from build123d import *

# Parameters (mm, degrees)
F0_W     = 101.6
F0_H     = 76.2
F0_W_2   = 95.25
F0_H_2   = 69.85
F1_DEPTH = 130
F2_W     = 250
F2_H     = 35
F3_DEPTH = 3.175


with BuildPart() as f1:
    # F0 (on Right) → F1 (new body, symmetric)
    with BuildSketch(Plane.YZ):
        Rectangle(F0_W, F0_H)
        Rectangle(F0_W_2, F0_H_2, mode=Mode.SUBTRACT)
    extrude(amount=F1_DEPTH, both=True)

    # F2 (on face) → F3 (cut, through all)
    with BuildSketch(Plane.XZ.offset(50.8)):
        with Locations((0, -15.6)):
            Rectangle(F2_W, F2_H)
    extrude(amount=-F3_DEPTH, mode=Mode.SUBTRACT)


solid = f1.part
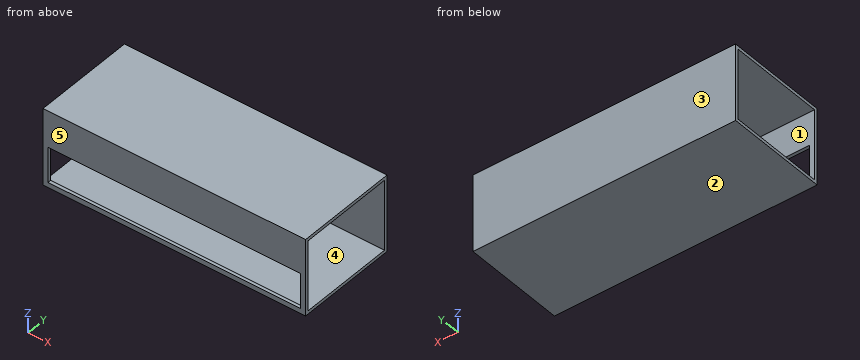
The model under review builds one solid part; all positions refer to its coordinate system, in mm. Face numbers are marked on the shaded views. A direction names the side the tool comes from. Coordinates: 2 decimals unless noted, no trailing zeros. Write each loop counter-clockwise with the first axis right and the second up, starting at its lowest first coordinate (ties: lowest second). Pieces come first, ordered by that corner, then holes. Notation, with made-up numbers: (72.25, 15) - (109.25, 15) arc R35 ccw to (109.25, 52) - close; hole circle Ø9 at (-27.75, -4). An arc over 180 degrees is marked (long way). Answer as a JSON object with one key per item and string values. Group by question number.
1. Add section A-A (z = -16). Give the boundary of the cut face in (x, y) (3 decimals), plus the area to 3 significant figures.
2. Add section D-D (x = 13). Give the boundary of the cut face in (y, z) (3 decimals), plus the area to 3 significant figures.
3. Clearance check with a flat-ended pin moving along its axis: pin 1 Ø10 at (x, z) = (-40.5, -24) entering from -Y (3 decimals). State where the tip first meets the part, or that it passes through.
4. Machinability: for the marked faces 4 and 5, which of the approach directions +Z, -Z, +X, -X, +Y, -Y give a long, thin tool a straight path to every point of the face, cutting with its end or side? Answer none if there is none.
5. To check wall thickness, follow probe 1 along Z at (x, y) = (-11, 14.5) (3 decimals); probe 2 along Y at (x, z) = (-26.5, 15) (3 decimals); probe 3 along Y at (x, z) = (17, -15) (3 decimals). State the ranges of each line that lie inside material, in increasing order.
6. Mouldability with a two-part tool opening along Y and no side actions: class the marked faces 1, 2 and 3 as pulls with the +Y half, pulls with the -Y half, needs draft (parallel to the pull), parting line crosses it, or undercut.
7. Add section B-B (y = -23.5). Give the boundary of the cut face in (x, z) (3 decimals), plus the area to 3 significant figures.
8. Add section C-C (z = 20.5). Give the boundary of the cut face in (x, y) (3 decimals).
Findings:
{
 "1": {"outline": "(-130, -50.8) - (-125, -50.8) - (-125, -47.625) - (-130, -47.625) - close; (-130, 47.625) - (130, 47.625) - (130, 50.8) - (-130, 50.8) - close; (125, -50.8) - (130, -50.8) - (130, -47.625) - (125, -47.625) - close", "area": "857 mm²"},
 "2": {"outline": "(-50.8, -38.1) - (50.8, -38.1) - (50.8, 38.1) - (-50.8, 38.1) - (-50.8, 1.9) - (-47.625, 1.9) - (-47.625, 34.925) - (47.625, 34.925) - (47.625, -34.925) - (-47.625, -34.925) - (-47.625, -33.1) - (-50.8, -33.1) - close", "area": "978 mm²"},
 "3": {"pin 1": "y = 47.625"},
 "4": {"face 4": "+X, -X", "face 5": "+Z, -Z, +X, -X, -Y"},
 "5": {"probe 1": "-38.1 to -34.925, 34.925 to 38.1", "probe 2": "-50.8 to -47.625, 47.625 to 50.8", "probe 3": "47.625 to 50.8"},
 "6": {"face 1": "undercut", "face 2": "needs draft", "face 3": "pulls with the +Y half"},
 "7": {"outline": "(-130, -38.1) - (130, -38.1) - (130, -34.925) - (-130, -34.925) - close; (-130, 34.925) - (130, 34.925) - (130, 38.1) - (-130, 38.1) - close", "area": "1,650 mm²"},
 "8": {"outline": "(-130, -50.8) - (130, -50.8) - (130, -47.625) - (-130, -47.625) - close; (-130, 47.625) - (130, 47.625) - (130, 50.8) - (-130, 50.8) - close"}
}
